Read the model definition and answer for the solid it produces. Units are mm, in the model's axes. A direction names the side the tool comes from. Round coordinates to 2 decimals unless told otherwise and drop trailing zeros. Order: outer loops, then holes, each group sorted by start corner. A loop starts at its lowest first (then second) coordinate and runs counter-clockwise, first axis right, second up. Notation, with made-up numbers: (89, -34) - (106, -34) arc R12 cw to (106, -29) - close; hole circle Ø5 at (38, 25.25). An arc over 180 degrees is marked (long way). Put each result on its own line as item: value. Start each with the question number.
Q1. Section A-A on z = 7.25 is taken. Give the vertices of the cut face in (x, y).
Q2. Find the intervals of material crossed by line 1 along Z through (x, y) = (0, 5); line 2 along Y through (x, z) = (-1.25, 6); line 3 along Y through (x, z) = (4, 2.25), in increasing order. Write a range as from..to.
Q3. Which of the six approach directions +Z, -Z, +X, -X, +Y, -Y give full straight-line access (tool end or side, diameter ignored) to faces 5 (the face through (-1, -13, 2.15)), 6 (the face through (0, -5.25, 10)), 7 (the face through (0, -7, 3.15)), 8 (the face through (0, 7, 2)), 9 (the face through (7, -1.95, 10))?
Q4. Each of these flat-tipped pins is pushed along its axis until it touches: pin 1 Ø2.5 at (y, z) = (-19, 1) entering from +X; pin 2 Ø0.8 at (x, y) = (0, -7) entering from -Z; pin 3 Ø2 at (y, z) = (5, 13.5) entering from -X. Where does it stop, or does it pass through?
Q5. Section B-B on y = 14.5 is taken. Give the vertices of the cut face in (x, z), then the cut area to 3 significant figures.
Q6. For a pull along Y with two mould halves and no side action, classify faces 1 (the face through (5.8, -4, 10)), 2 (the face through (-3.63, -22.45, 1.06)), 3 (the face through (-0.1, -6.25, 2.6)), 4 (the face through (-1, -3.25, 10)) as pulls with the +Y half, pulls with the -Y half, needs draft (parallel to the pull), parting line crosses it, or undercut.
Q7. Section C-C on x = -3 is taken. Give the vertices of the cut face in (y, z), then the cut area to 3 significant figures.
from build123d import *

# Parameters (mm, degrees)
SALIENTE_EXTRUIR1_DEPTH = 19.3
CROQUIS2_W              = 15.3
CROQUIS2_H              = 26.3
CORTAR_EXTRUIR1_DEPTH   = 9.3
CORTAR_EXTRUIR2_DEPTH   = 12
CROQUIS5_R              = 0.75
SALIENTE_EXTRUIR2_DEPTH = 2
CROQUIS6_W              = 19.3
CROQUIS6_H              = 25
SALIENTE_EXTRUIR3_DEPTH = 3


with BuildPart() as part:
    # Croquis1 → Saliente-Extruir1 (new body)
    with BuildSketch(Plane.XY):
        with BuildLine():
            Line((5.8, 23.05), (2.4, 23.05))
            Line((2.4, 23.05), (-5.8, -0.85))
            Line((-5.8, -0.85), (-5.8, -10.609737321))
            ThreePointArc((-5.8, -10.609737321), (-5.505459406, -11.318487649), (-4.795345946, -11.609726491))
            Line((-4.795345946, -11.609726491), (-4.702327027, -11.609293571))
            ThreePointArc((-4.702327027, -11.609293571), (-4.347270297, -11.754912992), (-4.2, -12.109288156))
            Line((-4.2, -12.109288156), (-4.2, -21.05))
            ThreePointArc((-4.2, -21.05), (-3.614213562, -22.464213562), (-2.2, -23.05))
            Line((-2.2, -23.05), (-0.2, -23.05))
            ThreePointArc((-0.2, -23.05), (1.214213562, -22.464213562), (1.8, -21.05))
            Line((1.8, -21.05), (1.8, -13.106955688))
            ThreePointArc((1.8, -13.106955688), (2.239339828, -12.046295517), (3.3, -11.606955688))
            Line((3.3, -11.606955688), (3.8, -11.606955688))
            ThreePointArc((3.8, -11.606955688), (5.214213562, -11.021169251), (5.8, -9.606955688))
            Line((5.8, -9.606955688), (5.8, 23.05))
        make_face()
    extrude(amount=SALIENTE_EXTRUIR1_DEPTH)

    # Croquis2 → Cortar-Extruir1 (cut)
    with BuildSketch(Plane.ZY.offset(5.8)):
        with Locations((9.65, 9.9)):
            Rectangle(CROQUIS2_W, CROQUIS2_H)
    extrude(amount=-CORTAR_EXTRUIR1_DEPTH, mode=Mode.SUBTRACT)

    # Croquis4 → Cortar-Extruir2 (cut)
    with BuildSketch(Plane.ZY.offset(5.8)):
        Polygon((2.15, -5.25), (2.15, -6.25), (3.15, -6.25), (3.15, -7.25), (2.15, -7.25), (2.15, -23.25), (19.55, -23.25), (19.55, -7.25), (16.15, -7.25), (16.15, -6.25), (17.15, -6.25), (17.15, -5.25), align=None)
    extrude(amount=-CORTAR_EXTRUIR2_DEPTH, mode=Mode.SUBTRACT)

    # Croquis5 → Saliente-Extruir2 (add)
    with BuildSketch(Plane(origin=(0, 0, 0), x_dir=(-1, 0, 0), z_dir=(0, 0, -1))):
        with Locations((0.885806677, -20.318206006)):
            Circle(CROQUIS5_R)
    extrude(amount=SALIENTE_EXTRUIR2_DEPTH)

    # Croquis6 → Saliente-Extruir3 (add)
    with BuildSketch(Plane(origin=(5.8, 0, 0), x_dir=(0, 0, -1), z_dir=(1, 0, 0))):
        with Locations((-9.65, 10.55)):
            Rectangle(CROQUIS6_W, CROQUIS6_H)
    extrude(amount=SALIENTE_EXTRUIR3_DEPTH)


solid = part.part
Findings:
1. outline: (-5.8, -5.25) - (5.8, -5.25) - (5.8, -1.95) - (8.8, -1.95) - (8.8, 23.05) - (3.5, 23.05) - (3.5, -3.25) - (-5.8, -3.25) - close
2. line 1: 0..2, 17.3..19.3
2. line 2: -5.25..-3.25
2. line 3: -7.25..-6.25, -5.25..23.05
3. face 5: +Z, +X, -X, -Y
3. face 6: +X, -X
3. face 7: +X, -X, -Y
3. face 8: -X, +Y
3. face 9: +Z, -Z, +X, -Y
4. pin 1: x = 1.8
4. pin 2: z = 0
4. pin 3: x = 3.5
5. outline: (-0.53, 0) - (8.8, 0) - (8.8, 19.3) - (-0.53, 19.3) - (-0.53, 17.3) - (3.5, 17.3) - (3.5, 2) - (-0.53, 2) - close
5. area: 118 mm2
6. face 1: needs draft
6. face 2: pulls with the -Y half
6. face 3: undercut
6. face 4: pulls with the +Y half
7. outline: (-22.88, 0) - (7.31, 0) - (7.31, 2) - (-3.25, 2) - (-3.25, 17.3) - (7.31, 17.3) - (7.31, 19.3) - (-7.25, 19.3) - (-7.25, 16.15) - (-6.25, 16.15) - (-6.25, 17.15) - (-5.25, 17.15) - (-5.25, 2.15) - (-6.25, 2.15) - (-6.25, 3.15) - (-7.25, 3.15) - (-7.25, 2.15) - (-22.88, 2.15) - close
7. area: 125 mm2
